from build123d import *

# Parameters (mm, degrees)
SKETCH1_W           = 345
SKETCH1_H           = 70
BOSS_EXTRUDE1_DEPTH = 5
SKETCH2_W           = 345
SKETCH2_H           = 5
BOSS_EXTRUDE2_DEPTH = 5
SKETCH3_W           = 75
SKETCH3_H           = 5
CUT_EXTRUDE1_DEPTH  = 5
SKETCH4_R           = 0.4
CUT_EXTRUDE2_DEPTH  = 5


with BuildPart() as part:
    # Sketch1 → Boss-Extrude1 (new body)
    with BuildSketch(Plane(origin=(0, 0, 0), x_dir=(1, 0, 0), z_dir=(0, 1, 0))):
        with Locations((172.5, 35)):
            Rectangle(SKETCH1_W, SKETCH1_H)
    extrude(amount=BOSS_EXTRUDE1_DEPTH)

    # Sketch2 → Boss-Extrude2 (add)
    with BuildSketch(Plane(origin=(0, 5, 0), x_dir=(1, 0, 0), z_dir=(0, 1, 0))):
        with Locations((172.5, 67.5)):
            Rectangle(SKETCH2_W, SKETCH2_H)
        with Locations((172.5, 2.5)):
            Rectangle(SKETCH2_W, SKETCH2_H)
    extrude(amount=BOSS_EXTRUDE2_DEPTH)

    # Sketch3 → Cut-Extrude1 (cut)
    with BuildSketch(Plane(origin=(0, 10, 0), x_dir=(1, 0, 0), z_dir=(0, 1, 0))):
        with Locations((172.5, 2.5)):
            Rectangle(SKETCH3_W, SKETCH3_H)
    extrude(amount=-CUT_EXTRUDE1_DEPTH, mode=Mode.SUBTRACT)

    # Sketch4 → Cut-Extrude2 (cut)
    with BuildSketch(Plane(origin=(0, 0, -70), x_dir=(-1, 0, 0), z_dir=(0, 0, -1))):
        with Locations((-335.6, 5)):
            Circle(SKETCH4_R)
        with Locations((-260.2, 5)):
            Circle(SKETCH4_R)
        with Locations((-184.8, 5)):
            Circle(SKETCH4_R)
        with Locations((-109.4, 5)):
            Circle(SKETCH4_R)
        with Locations((-34, 5)):
            Circle(SKETCH4_R)
    extrude(amount=-CUT_EXTRUDE2_DEPTH, mode=Mode.SUBTRACT)


solid = part.part
Verification items for the finished model (mm, model axes). Round coordinates to 2 decimals unless told otherwise and drop trailing zeros. Write each loop counter-clockwise with the first axis right and the second up, starting at its lowest first coordinate (ties: lowest second). Pieces come first, ordered by that corner, then holes.
(1) Section check A-A (y = 8). Enter the section's corners in (x, z).
Returned:
outline: (0, -70) - (345, -70) - (345, -65) - (0, -65) - close; (0, -5) - (135, -5) - (135, 0) - (0, 0) - close; (210, -5) - (345, -5) - (345, 0) - (210, 0) - close
(2) Section check B-B (x = 303). Enter the section's corners in (y, z).
Returned:
outline: (0, -70) - (10, -70) - (10, -65) - (5, -65) - (5, -5) - (10, -5) - (10, 0) - (0, 0) - close
(3) Material ranges on line 1 (Y direction, x = 184.8, z = -66.25); line 2 (Z direction, x = 265.5, y = 5.5); line 3 (Y direction, x = 43, z = -38), recorded low to high.
Returned:
line 1: y = 0 to 4.6, 5.4 to 10
line 2: z = -70 to -65, -5 to 0
line 3: y = 0 to 5
(4) Depth check by flat-ended pin: pin 1 Ø10 at (x, z) = (258.5, -10.5) entering from +Y; pin 2 Ø10 at (x, z) = (180.5, -56) entering from -Y; pin 3 Ø5.5 at (x, y) = (176, 8.5) entering from +Z. Enter the tip coordinate at first touch or a pass-through.
Returned:
pin 1: stops at y = 5
pin 2: stops at y = 0
pin 3: stops at z = -65
